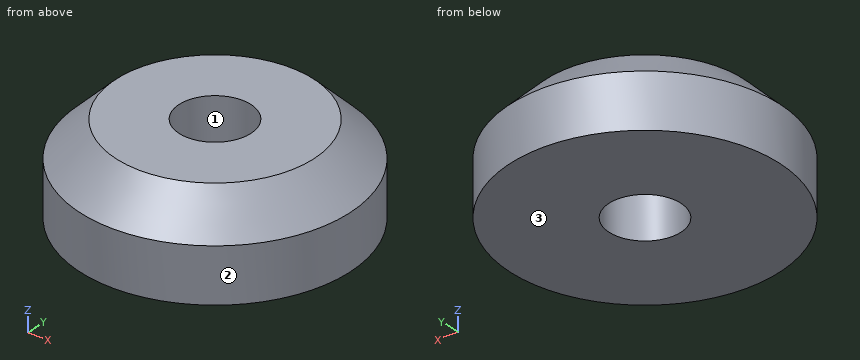
```python
from build123d import *

# Parameters (mm, degrees)
F0_R     = 7.5
F1_DEPTH = 5
F2_R     = 2
F3_DEPTH = 25
F4_SIZE  = 2


with BuildPart() as f1:
    # F0 (on Top) → F1 (new body)
    with BuildSketch(Plane.XY):
        Circle(F0_R)
    extrude(amount=F1_DEPTH)

    # F2 (on face) → F3 (cut)
    with BuildSketch(Plane.XY.offset(5)):
        Circle(F2_R)
    extrude(amount=-F3_DEPTH, mode=Mode.SUBTRACT)

    # F4
    f4_edges = [f1.edges().sort_by_distance(p)[0] for p in [
        (-7.5, 0, 5),
    ]]
    chamfer(f4_edges, length=F4_SIZE)


solid = f1.part
```
Here's how the part is built. I have some questions about the finished solid (model axes, mm). Face numbers are marked on the shaded views. Coordinates: 2 decimals unless noted, no trailing zeros. Loops run counter-clockwise (first coordinate to the right, second up) from the corner with the lowest first, then second, coordinate; pieces in that order, holes last. Notation, with made-up numbers: (12.25, 12.25) - (21.25, 12.25) arc R22 cw to (21.25, 31.25) - close; hole circle Ø5 at (39, 41). An arc over 180 degrees is marked (long way). Return JSON: item names as keys, results as strings. Group by question number.
Item 1: Will these pins go through, and if not, where does the flat tip stop? P1, Ø1.5, axis at x = -1.5, z = 3, coming from the +Y side; P2, Ø2, axis at y = 4.5, z = 3, coming from the +X side; P3, Ø1, axis at x = 2.5, z = 4.5, coming from the +Y side.
Item 2: I need wall thicknesses on line 1 (Y direction, x = 0, z = 1.35); line 2 (Y direction, x = 1.5, z = 2.8); line 3 (X direction, y = 0.5, z = 3.35). Which ranges of each line are inside material? Lowest first, please. Write a range as from..to.
Item 3: If we section it at A-A on y = 0: Write out the boundary of the cut face in (x, z).
Item 4: If we section it at C-C on z = 0.4: Write out the boundary of the cut face in (x, y), and give its area (3 significant figures).
Item 5: We'd pull the mould along X, two halves only. Please class the marked faces 1, 2 and 3: +X half, -X half, draft (parallel to the pull), parting line (faces both ways), or undercut.
Calculated:
{
 "1": {"P1": "stops at y = 7.46", "P2": "stops at x = 6.63", "P3": "stops at y = 6.04"},
 "2": {"line 1": "y = -7.5..-2, 2..7.5", "line 2": "y = -7.35..-1.32, 1.32..7.35", "line 3": "x = -7.13..-1.94, 1.94..7.13"},
 "3": {"outline": "(-7.5, 0) - (-2, 0) - (-2, 5) - (-5.5, 5) - (-7.5, 3) - close; (2, 0) - (7.5, 0) - (7.5, 3) - (5.5, 5) - (2, 5) - close"},
 "4": {"outline": "circle Ø15 at (0, 0); hole circle Ø4 at (0, 0)", "area": "164 mm^2"},
 "5": {"face 1": "undercut", "face 2": "parting line", "face 3": "draft"}
}
